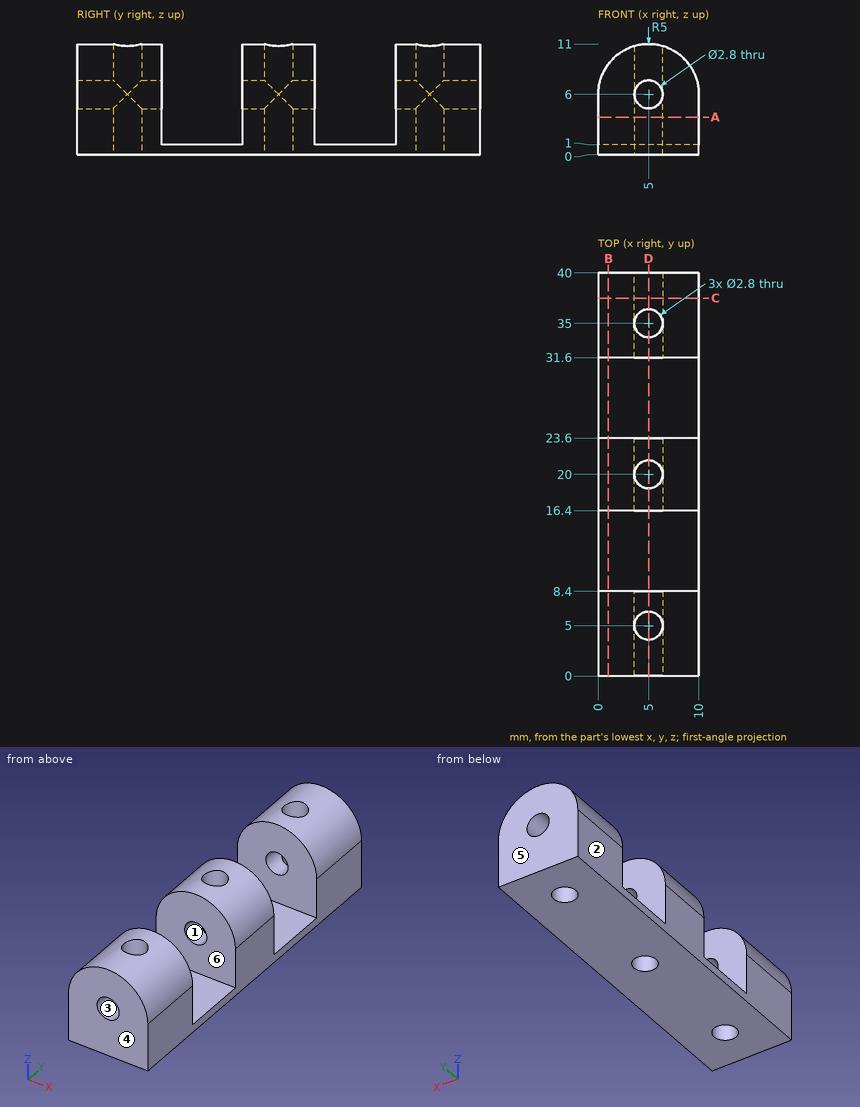
Input: dimensioned drawing with shaded views. Units: mm. Origin: part minimum x, y, z. A direction names the side the tool comes from. Give positions to 0.01 mm unless a question says otherwise; leave off trailing zeros. Write each loop counter-clockwise with the first axis right and the second up, starting at its lowest first coordinate (ties: lowest second). Pieces come first, ordered by that corner, then holes. Notation, with made-up numbers: (72.25, 34.25) -> (116.25, 34.25) arc R16 ccw to (116.25, 64.25) -> close; hole circle Ø8 at (74.25, -25.75). An arc over 180 degrees is marked (long way). Answer as a JSON object with one key per item and string values.
1. Cut plane B-B on x = 1. Output: boundary loops of the cut face in (y, z), and give its area (3 significant figures).
Ans:
{"outline": "(0, 0) -> (40, 0) -> (40, 9) -> (31.6, 9) -> (31.6, 1) -> (23.6, 1) -> (23.6, 9) -> (16.4, 9) -> (16.4, 1) -> (8.4, 1) -> (8.4, 9) -> (0, 9) -> close", "area": "232 mm^2"}
2. Ray query, probe 1 along Y at (x, z) = (2, 9); probe 2 along X at (y, z) = (36.1, 6); probe 3 along Y at (x, z) = (5, 9.7). Return the intervals inside material, ascending. Write a range as from..to.
Ans:
{"probe 1": "y = 0..8.4, 16.4..23.6, 31.6..40", "probe 2": "x = 0..3.6, 6.4..10", "probe 3": "y = 0..3.6, 6.4..8.4, 16.4..18.6, 21.4..23.6, 31.6..33.6, 36.4..40"}
3. Mould query, pull axis X, two halves, no side actions, for the marked faces 1, 2, 3 and 4. Classes: pulls with the +X half, pulls with the -X half, needs draft (parallel to the pull), parting line crosses it, or undercut.
Ans:
{"face 1": "undercut", "face 2": "pulls with the -X half", "face 3": "undercut", "face 4": "needs draft"}
4. Access query for the marked faces 5 and 6. Directions: +Z, -Z, +X, -X, +Y, -Y. A direction counts if a zero-diameter tool reaches every point of the face in a straight line with its end or side. Return the directions, or none.
Ans:
{"face 5": "+Z, -Z, +X, -X, +Y", "face 6": "+Z, +X, -X"}
5. Cut plane A-A on z = 3.75. Output: boundary loops of the cut face in (x, y), and give its area (3 significant figures).
Ans:
{"outline": "(0, 0) -> (10, 0) -> (10, 8.4) -> (0, 8.4) -> close; (0, 16.4) -> (10, 16.4) -> (10, 23.6) -> (0, 23.6) -> close; (0, 31.6) -> (10, 31.6) -> (10, 40) -> (0, 40) -> close; hole circle Ø2.8 at (5, 5); hole circle Ø2.8 at (5, 20); hole circle Ø2.8 at (5, 35)", "area": "222 mm^2"}
6. Cut plane C-C on y = 37.5. Output: boundary loops of the cut face in (x, z), and give its area (3 significant figures).
Ans:
{"outline": "(0, 0) -> (10, 0) -> (10, 6) arc R5 ccw to (0, 6) -> close; hole circle Ø2.8 at (5, 6)", "area": "93.1 mm^2"}
7. Contact query for a flat-ended pin moving along its axis: pin 1 (1 mm diameter, centred on x = 5, y = 26.5, fed in from +Z). Output: stop coordinate, or through.
Ans:
{"pin 1": "stops at z = 1"}
8. Cut plane D-D on x = 5. Count the separate pieces of the cut face and the enclosed holes in it, and give its area (3 significant figures).
Ans:
{"separate pieces": "10", "enclosed holes": "0", "area": "144 mm^2"}
